from build123d import *

# Parameters (mm, degrees)
SKETCH_1_W          = 60
SKETCH_1_H          = 20
EXTRUDE_1_DEPTH     = 6
FILLET_1_R          = 2
SKETCH_2_R          = 2.2
CUT_EXTRUDE_1_DEPTH = 33.186953879
CUT_EXTRUDE_2_DEPTH = 33.186953879


with BuildPart() as part:
    # 草图1 → 凸台-拉伸1 (new body)
    with BuildSketch(Plane.XY):
        Rectangle(SKETCH_1_W, SKETCH_1_H)
    extrude(amount=EXTRUDE_1_DEPTH)

    # 圆角1
    fillet_1_edges = [part.edges().sort_by_distance(p)[0] for p in [
        (30, -10, 3),
        (-30, -10, 3),
        (-30, 10, 3),
        (30, 10, 3),
    ]]
    fillet(fillet_1_edges, radius=FILLET_1_R)

    # 草图2 → 切除-拉伸1 (cut, through all)
    with BuildSketch(Plane.XY.offset(6)):
        with Locations((22.5, 0)):
            Circle(SKETCH_2_R)
        with Locations((7.5, 0)):
            Circle(SKETCH_2_R)
    extrude(amount=-CUT_EXTRUDE_1_DEPTH, mode=Mode.SUBTRACT)

    # 草图3 → 切除-拉伸2 (cut, through all)
    with BuildSketch(Plane.XY.offset(6)):
        with BuildLine():
            Line((-19.5, 7), (-4.5, 7))
            ThreePointArc((-4.5, 7), (2.5, 0), (-4.5, -7))
            Line((-4.5, -7), (-19.5, -7))
            ThreePointArc((-19.5, -7), (-26.5, 0), (-19.5, 7))
        make_face()
        with BuildLine():
            Line((12.5, -5), (12.5, 5))
            ThreePointArc((12.5, 5), (15, 7.5), (17.5, 5))
            Line((17.5, 5), (17.5, -5))
            ThreePointArc((17.5, -5), (15, -7.5), (12.5, -5))
        make_face()
    extrude(amount=-CUT_EXTRUDE_2_DEPTH, mode=Mode.SUBTRACT)


solid = part.part
CAD build for the part. Positions are in the model's coordinates, mm. A direction names the side the tool comes from. Round coordinates to 2 decimals unless told otherwise and drop trailing zeros. Write each loop counter-clockwise with the first axis right and the second up, starting at its lowest first coordinate (ties: lowest second). Pieces come first, ordered by that corner, then holes.
(1) Mould opens along X. For faces 1 (the face through (6, 2, 6)), 2 (the face through (24.532, -0.843, 3.042)), 3 (the face through (17.5, 0, 3)), 4 (the face through (29.43, 9.4, 3.04)) say: pulls with the +X half, pulls with the -X half, needs draft (parallel to the pull), parting line crosses it, or undercut.
(2) 3-axis set-ups, long thin cutter, end or side, ignore diameter. For faces 5 (the face through (15.1, -7.5, 3)), 6 (the face through (0, 10, 3)): which of +Z, -Z, +X, -X, +Y, -Y reach the whole face in a straight line?
(3) Slice it at B-B, the plane y = 0. Write the cut outline in (x, z).
(4) Slice it at A-A, the plane x = 15. Write the cut outline in (y, z).
(5) Probe line 1 along X through (y, z) = (-3.5, 3.4); line 2 along X through (y, z) = (2.5, 2.25); line 3 along Y through (x, z) = (-15.5, 1.55). List the from-to ranges inside material, lowest first.
(6) Slice it at D-D, the plane y = 3.25. Write the cut outline in (x, z), and give its area (3 significant figures).
(7) Slice it at C-C, the plane z = 0.75. Write the cut outline in (x, y), and give its area (3 significant figures).
From the geometry:
1. face 1: needs draft
1. face 2: undercut
1. face 3: undercut
1. face 4: pulls with the +X half
2. face 5: +Z, -Z
2. face 6: +Z, -Z, +X, -X, +Y
3. outline: (-30, 0) - (-26.5, 0) - (-26.5, 6) - (-30, 6) - close; (2.5, 0) - (5.3, 0) - (5.3, 6) - (2.5, 6) - close; (9.7, 0) - (12.5, 0) - (12.5, 6) - (9.7, 6) - close; (17.5, 0) - (20.3, 0) - (20.3, 6) - (17.5, 6) - close; (24.7, 0) - (30, 0) - (30, 6) - (24.7, 6) - close
4. outline: (-10, 0) - (-7.5, 0) - (-7.5, 6) - (-10, 6) - close; (7.5, 0) - (10, 0) - (10, 6) - (7.5, 6) - close
5. line 1: x = -30 to -25.56, 1.56 to 12.5, 17.5 to 30
5. line 2: x = -30 to -26.04, 2.04 to 12.5, 17.5 to 30
5. line 3: y = -10 to -7, 7 to 10
6. outline: (-30, 0) - (-25.7, 0) - (-25.7, 6) - (-30, 6) - close; (1.7, 0) - (12.5, 0) - (12.5, 6) - (1.7, 6) - close; (17.5, 0) - (30, 0) - (30, 6) - (17.5, 6) - close
6. area: 166 mm2
7. outline: (-30, -8) arc R2 ccw to (-28, -10) - (28, -10) arc R2 ccw to (30, -8) - (30, 8) arc R2 ccw to (28, 10) - (-28, 10) arc R2 ccw to (-30, 8) - close; hole (-19.5, -7) - (-4.5, -7) arc R7 ccw to (-4.5, 7) - (-19.5, 7) arc R7 ccw to start; hole circle Ø4.4 at (7.5, 0); hole (12.5, -5) arc R2.5 ccw to (17.5, -5) - (17.5, 5) arc R2.5 ccw to (12.5, 5) - close; hole circle Ø4.4 at (22.5, 0)
7. area: 733 mm2
